```python
from build123d import *

# Parameters (mm, degrees)
F0_R        = 2
F1_DEPTH    = 3.175
F2_R        = 5
F3_R        = 2
F4_W        = 3
F4_H        = 24
F5_DEPTH    = 1
F6_T1_DEPTH = 24


# Not quite as in the source:
# - a fillet or chamfer that OpenCascade refuses, or shapes differently, is made with other operations: its cross-section is extruded or revolved along the edge and cut away or added


with BuildPart() as f1:
    # F0 (on Top) → F1 (new body)
    with BuildSketch(Plane.XY):
        with BuildLine():
            Line((11.2449979984, 0), (0, 0))
            Line((0, 0), (0, 11.2449979984))
            ThreePointArc((0, 11.2449979984), (-0.6568542495, -0.6568542495), (11.2449979984, 0))
        make_face()
        Polygon((0, 11.2449979984), (0, 0), (11.2449979984, 0), (41, 0), (70.7550020016, 0), (82, 0), (82, 11.2449979984), (82, 24), (57.1, 24), (57.1, 19), (41, 19), (24.9, 19), (24.9, 24), (0, 24), align=None)
        with Locations((5, 5)):
            Circle(F0_R, mode=Mode.SUBTRACT)
        with Locations((77, 5)):
            Circle(F0_R, mode=Mode.SUBTRACT)
        with BuildLine():
            Line((82, 0), (70.7550020016, 0))
            ThreePointArc((70.7550020016, 0), (82.6568542495, -0.6568542495), (82, 11.2449979984))
            Line((82, 11.2449979984), (82, 0))
        make_face()
    extrude(amount=F1_DEPTH)

    # F2
    f2_edges = [f1.edges().sort_by_distance(p)[0] for p in [
        (11.244998, 0, 1.5875),
        (70.755002, 0, 1.5875),
        (82, 11.244998, 1.5875),
        (0, 11.244998, 1.5875),
    ]]
    fillet(f2_edges, radius=F2_R)

    # F3
    f3_edges = [f1.edges().sort_by_distance(p)[0] for p in [
        (24.9, 19, 1.5875),
        (57.1, 19, 1.5875),
    ]]
    fillet(f3_edges, radius=F3_R)

    # F4 (on face) → F5 (join)
    with BuildSketch(Plane.XY.offset(3.175)):
        with Locations((20.4, 12)):
            Rectangle(F4_W, F4_H)
        with Locations((61.6, 12)):
            Rectangle(F4_W, F4_H)
    extrude(amount=F5_DEPTH)

    # F6: fillet of radius 5 on 4 edges, made by hand

    # F6_s2 → F6_t1 (join)
    with BuildSketch(Plane.XZ.offset(-24)):
        with BuildLine():
            ThreePointArc((15.9, 3.175), (17.4811388301, 3.4315835097), (18.9, 4.175))
            Line((18.9, 4.175), (18.96, 4.095))
            ThreePointArc((18.96, 4.095), (19, 3.675), (19, 3.175))
            Line((19, 3.175), (18.9, 3.075))
            Line((18.9, 3.075), (15.9, 3.075))
            Line((15.9, 3.075), (15.9, 3.175))
        make_face()
        with BuildLine():
            ThreePointArc((24.9, 3.175), (23.3188611699, 3.4315835097), (21.9, 4.175))
            Line((21.9, 4.175), (21.84, 4.095))
            ThreePointArc((21.84, 4.095), (21.8, 3.675), (21.8, 3.175))
            Line((21.8, 3.175), (21.9, 3.075))
            Line((21.9, 3.075), (24.9, 3.075))
            Line((24.9, 3.075), (24.9, 3.175))
        make_face()
        with BuildLine():
            ThreePointArc((57.1, 3.175), (58.6811388301, 3.4315835097), (60.1, 4.175))
            Line((60.1, 4.175), (60.16, 4.095))
            ThreePointArc((60.16, 4.095), (60.2, 3.675), (60.2, 3.175))
            Line((60.2, 3.175), (60.1, 3.075))
            Line((60.1, 3.075), (57.1, 3.075))
            Line((57.1, 3.075), (57.1, 3.175))
        make_face()
        with BuildLine():
            ThreePointArc((66.1, 3.175), (64.5188611699, 3.4315835097), (63.1, 4.175))
            Line((63.1, 4.175), (63.04, 4.095))
            ThreePointArc((63.04, 4.095), (63, 3.675), (63, 3.175))
            Line((63, 3.175), (63.1, 3.075))
            Line((63.1, 3.075), (66.1, 3.075))
            Line((66.1, 3.075), (66.1, 3.175))
        make_face()
    extrude(amount=F6_T1_DEPTH)


solid = f1.part
```
Check sheet for the modelled part. Datum: model origin and axes. Units: mm. A direction names the side the tool comes from. Give positions to 0.01 mm unless a question says otherwise; leave off trailing zeros. Order: outer loops, then holes, each group sorted by start corner. A loop starts at its lowest first (then second) coordinate and runs counter-clockwise, first axis right, second up. Notation, with made-up numbers: M -40,16.25 L -3,16.25 A26 cw -3,43.25 Z; hole C 51,2 d1. An arc over 180 degrees is marked long. Answer in a Markdown table with one row per item. Add a question column.
Q1. Access from +Z, -Z, +X, -X, +Y, -Y to the whole of each face (thin tool, end or side, straight path). Record for faces 1 (the flat face through (75, 11, 3.175)), 2 (the flat face through (0, 19, 2)), 3 (the flat face through (41, 11, 3.175)), 4 (the cylindrical face through (25.47, 19.6, 1.61)).
Q2. Gauge pin test, flat ends, axial feed: pin 1 Ø2 at (y, z) = (8, 3) entering from -X; pin 2 Ø15 at (x, y) = (5.5, 10.5) entering from +Z (3 decimals); pin 3 Ø1 at (y, z) = (17.5, 2) entering from +X. Record the tip position at first contact, or that the pin passes through.
Q3. Sectioned sample at C-C, the plane y = 5. Record the boundary of the cut face in (x, z) (3 decimals).
Q4. Release check for a two-part mould opening along Y. For faces 5 (the flat face through (41, 19, 2)), 6 (the cylindrical face through (3, 5, 2)), 7 (the cylindrical face through (17.46, 12.168, 3.425)), 8 (the cylindrical face through (11.6, -0.3, 1.6)) record: released by +Y, released by -Y, zero draft, split by the parting line, or undercut.
Q5. Sectioned sample at D-D, the plane x = 30. Record the boundary of the cut face in (y, z) (3 decimals).
Q6. Sectioned sample at A-A, the plane x = 5. Record the boundary of the cut face in (y, z) (3 decimals).
Q7. Thickness scan on L1, parallel to Y at x = 77, z = 1.15; L2, parallel to X at y = 17.75, z = 2.65; L3, parallel to Y at x = 47.5, z = 1. Record the ranges inside material, lowest first.
Q8. Sectioned sample at B-B, the plane z = 2.4. Record the boundary of the cut face in (x, y).
Verdict:
| question | item | result |
|---|---|---|
| 1 | face 1 | +Z, +X, +Y, -Y |
| 1 | face 2 | +Z, -Z, -X, +Y |
| 1 | face 3 | +Z, +Y, -Y |
| 1 | face 4 | +Z, -Z, +Y |
| 2 | pin 1 | x = -2.75 |
| 2 | pin 2 | z = 3.175 |
| 2 | pin 3 | x = 82 |
| 3 | outline | M -3,0 L 3,0 L 3,3.175 L -3,3.175 Z; M 7,0 L 75,0 L 75,3.175 L 66.1,3.175 A5 cw 63.1,4.175 L 60.1,4.175 A5 cw 57.1,3.175 L 24.9,3.175 A5 cw 21.9,4.175 L 18.9,4.175 A5 cw 15.9,3.175 L 7,3.175 Z; M 79,0 L 85,0 L 85,3.175 L 79,3.175 Z |
| 4 | face 5 | released by +Y |
| 4 | face 6 | undercut |
| 4 | face 7 | zero draft |
| 4 | face 8 | released by -Y |
| 5 | outline | M 0,0 L 19,0 L 19,3.175 L 0,3.175 Z |
| 6 | outline | M -3,0 L 3,0 L 3,3.175 L -3,3.175 Z; M 7,0 L 24,0 L 24,3.175 L 7,3.175 Z |
| 7 | L1 | -3 to 3, 7 to 24 |
| 7 | L2 | 0 to 82 |
| 7 | L3 | 0 to 19 |
| 8 | outline | M -1.15,10.11 A8 ccw 10.11,-1.15 A5 cw 13.31,0 L 68.69,0 A5 cw 71.89,-1.15 A8 ccw 83.15,10.11 A5 cw 82,13.31 L 82,24 L 57.1,24 L 57.1,21 A2 cw 55.1,19 L 26.9,19 A2 cw 24.9,21 L 24.9,24 L 0,24 L 0,13.31 A5 cw Z; hole C 5,5 d4; hole C 77,5 d4 |
